from build123d import *

# Parameters (mm, degrees)
BOSS_EXTRUDE1_DEPTH = 6.35
FILLET1_R           = 2.54


with BuildPart() as part:
    # Sketch1 → Boss-Extrude1 (new body)
    with BuildSketch(Plane.XY):
        Polygon((0, 0), (0, 15.875), (12.7, 15.875), (12.7, 20.6121), (-12.7, 20.6121), (-12.7, 0), align=None)
    extrude(amount=BOSS_EXTRUDE1_DEPTH)

    # Fillet1
    # the kernel refuses this fillet: 2.54 mm, written as the material it adds along each edge
    with BuildSketch(Plane(origin=(0, 15.875, 0), x_dir=(0, -1, 0), z_dir=(0, 0, 1))) as fillet1_piece_1:
        with BuildLine():
            CenterArc((FILLET1_R, FILLET1_R), FILLET1_R, 180, 90)
            Line((0, FILLET1_R), (0, 0))
            Line((0, 0), (FILLET1_R, 0))
        make_face()
    extrude(amount=6.35)
    # the kernel refuses this fillet: 2.54 mm, written as the material it takes off along each edge
    with BuildSketch(Plane(origin=(12.7, 15.875, -6.35), x_dir=(-1, 0, 0), z_dir=(0, 0, 1)), Plane(origin=(12.7, 20.6121, -6.35), x_dir=(0, -1, 0), z_dir=(0, 0, 1)), Plane(origin=(-12.7, 20.6121, -6.35), x_dir=(1, 0, 0), z_dir=(0, 0, 1))) as fillet1_2_piece_1:
        with BuildLine():
            CenterArc((FILLET1_R, -FILLET1_R), FILLET1_R, 90, 90)
            Line((0, -FILLET1_R), (0, 0))
            Line((0, 0), (FILLET1_R, 0))
        make_face()
    extrude(amount=19.05, mode=Mode.SUBTRACT)


solid = part.part
Can you work these out from the model? Positions are in its coordinate system, mm. A direction names the side the tool comes from. Coordinates: 2 decimals unless noted, no trailing zeros. Loops run counter-clockwise (first coordinate to the right, second up) from the corner with the lowest first, then second, coordinate; pieces in that order, holes last. Notation, with made-up numbers: (-20, 8.5) - (29, 8.5) arc R20 ccw to (29, 15.5) - close; hole circle Ø7 at (-36, 72). An arc over 180 degrees is marked (long way). Put each result on its own line as item: value. Start each with the question number.
Item 1: If I drill on line 1 along X through (y, z) = (13.5, 5.5); line 2 along Y through (x, z) = (3, 5.25) (3 decimals); line 3 along X through (y, z) = (18.25, 4.5), over which ranges is the centre line in solid material (lowest first)?
Item 2: Suppose I cut it at C-C (x = 3). Please give me the cut outline in (y, z) (3 decimals).
Item 3: Which directions (+Z, -Z, +X, -X, +Y, -Y) give clear straight access to the entire face, cutting with the end or side of a thin tool? Please do faces 1 (the face through (-6, 0, 3)), 2 (the face through (0, 7, 3)).
Item 4: Suppose I cut it at A-A (z = 1). Please give me the cut outline in (x, y) (3 decimals).
Item 5: For pin 1 (1.5 mm diameter, centred on y = 9.5, z = 2.5, fed in from +X); pin 2 (3 mm diameter, centred on x = 6.5, z = 5.5, fed in from -Y) (3 decimals), each with a flat end and sliding along its axis, tell me the tip position at first contact or that it passes through.
Item 6: Suppose I cut it at B-B (y = 4.25). Please give me the cut outline in (x, z).
Here are the results:
1. line 1: -12.7 to 0.01
1. line 2: 15.875 to 20.612
1. line 3: -12.69 to 12.69
2. outline: (15.875, 0) - (20.612, 0) - (20.612, 6.35) - (15.875, 6.35) - close
3. face 1: +Z, -Z, +X, -X, -Y
3. face 2: +Z, -Z, +X, -Y
4. outline: (-12.7, 0) - (0, 0) - (0, 13.335) arc R2.54 cw to (2.54, 15.875) - (10.16, 15.875) arc R2.54 ccw to (12.694, 18.244) arc R2.54 ccw to (10.16, 20.612) - (-10.16, 20.612) arc R2.54 ccw to (-12.7, 18.072) - close
5. pin 1: x = 0
5. pin 2: y = 15.875
6. outline: (-12.7, 0) - (0, 0) - (0, 6.35) - (-12.7, 6.35) - close
